```python
from build123d import *

# Parameters (mm, degrees)
SKETCH_1_W               = 35
SKETCH_1_H               = 25
EXTRUDE_1_DEPTH          = 8
FILLET_1_R               = 3
SKETCH_2_R               = 1.524999998
CUT_EXTRUDE_1_DEPTH      = 1
CUT_EXTRUDE_1_DEPTH_BACK = 9
SKETCH_3_R               = 3.099999998
CUT_EXTRUDE_2_DEPTH      = 4
HOLE_WIZARD_M4_1_D       = 3.3
HOLE_WIZARD_M4_2_D       = 3.3


with BuildPart() as part:
    # 草图1 → 凸台-拉伸1 (new body)
    with BuildSketch(Plane.XY):
        Rectangle(SKETCH_1_W, SKETCH_1_H)
    extrude(amount=EXTRUDE_1_DEPTH)

    # 圆角1
    fillet_1_edges = [part.edges().sort_by_distance(p)[0] for p in [
        (17.5, -12.5, 4),
        (-17.5, -12.5, 4),
        (-17.5, 12.5, 4),
        (17.5, 12.5, 4),
    ]]
    fillet(fillet_1_edges, radius=FILLET_1_R)

    # 草图2 → 切除-拉伸1 (cut, two sides)
    with BuildSketch(Plane.XY.offset(8)) as cut_extrude_1_sk:
        with Locations((3, 5.000000008)):
            Circle(SKETCH_2_R)
        with Locations((3, -4.999999992)):
            Circle(SKETCH_2_R)
        with Locations((-12, 5.000000008)):
            Circle(SKETCH_2_R)
        with Locations((-12, -4.999999992)):
            Circle(SKETCH_2_R)
    extrude(amount=CUT_EXTRUDE_1_DEPTH, mode=Mode.SUBTRACT)
    extrude(cut_extrude_1_sk.sketch, amount=-CUT_EXTRUDE_1_DEPTH_BACK, mode=Mode.SUBTRACT)

    # 草图3 → 切除-拉伸2 (cut)
    with BuildSketch(Plane.XY.offset(8)):
        with Locations((3, 5.000000008)):
            Circle(SKETCH_3_R)
        with Locations((-12, 5.000000008)):
            Circle(SKETCH_3_R)
        with Locations((3, -4.999999992)):
            Circle(SKETCH_3_R)
        with Locations((-12, -4.999999992)):
            Circle(SKETCH_3_R)
    extrude(amount=-CUT_EXTRUDE_2_DEPTH, mode=Mode.SUBTRACT)

    # M4 螺纹孔1 (through all)
    with Locations(Plane(origin=(-3.5, -12.5, 4), x_dir=(0, 0, -1), z_dir=(0, -1, 0))):
        with Locations((0, 0), (0, 15)):
            Hole(HOLE_WIZARD_M4_1_D / 2)

    # M4 螺纹孔2 (through all)
    with Locations(Plane.ZY.offset(17.5)):
        with Locations((4, 9e-09)):
            Hole(HOLE_WIZARD_M4_2_D / 2)


solid = part.part
```
For this review, take the finished solid that the model builds, in its own axes (mm). A direction names the side the tool comes from. Round coordinates to 2 decimals unless told otherwise and drop trailing zeros. Loops run counter-clockwise (first coordinate to the right, second up) from the corner with the lowest first, then second, coordinate; pieces in that order, holes last.
(1) Tool access review of faces 4 (the cylindrical face through (-15.1, -4.9, 6)), 5 (the flat face through (0, 0, 8)): name each direction out of +Z, -Z, +X, -X, +Y, -Y from which nothing blocks a thin tool from reaching the whole face with its end or side.
Returned:
face 4: +Z
face 5: +Z, +X, -X, +Y, -Y
(2) We need section B-B (x = 3). Give the boundary of the cut face in (y, z) (3 decimals), plus the area to 3 significant figures.
Returned:
outline: (-12.5, 0) - (-6.525, 0) - (-6.525, 4) - (-8.1, 4) - (-8.1, 8) - (-12.5, 8) - close; (-3.475, 0) - (3.475, 0) - (3.475, 4) - (1.9, 4) - (1.9, 8) - (-1.9, 8) - (-1.9, 4) - (-3.475, 4) - close; (6.525, 0) - (12.5, 0) - (12.5, 8) - (8.1, 8) - (8.1, 4) - (6.525, 4) - close; hole circle Ø3.3 at (0, 4)
area: 117 mm2
(3) We need section C-C (z = 4.75). State how many separate pieces and enclosed holes the cut face has, plus the area to 3 significant figures.
Returned:
separate pieces: 6
enclosed holes: 4
area: 514 mm2
(4) We need section A-A (y = 5). Give the boundary of the cut face in (x, z) (3 decimals), plus the area to 3 significant figures.
Returned:
outline: (-17.5, 0) - (-13.525, 0) - (-13.525, 4) - (-15.1, 4) - (-15.1, 8) - (-17.5, 8) - close; (-10.475, 0) - (1.475, 0) - (1.475, 4) - (-0.1, 4) - (-0.1, 8) - (-8.9, 8) - (-8.9, 4) - (-10.475, 4) - close; (4.525, 0) - (17.5, 0) - (17.5, 8) - (6.1, 8) - (6.1, 4) - (4.525, 4) - close; hole circle Ø3.3 at (-3.5, 4); hole circle Ø3.3 at (11.5, 4)
area: 189 mm2
(5) Wall thickness on line 1 along Y through (x, z) = (3, 5.75); line 2 along X through (y, z) = (11.25, 5.5); line 3 along X through (y, z) = (3.25, 3.75): over which ranges is each line inside the solid? List them lowest first.
Returned:
line 1: y = -12.5 to -8.1, -1.9 to 1.9, 8.1 to 12.5
line 2: x = -16.94 to -4.19, -2.81 to 10.81, 12.19 to 16.94
line 3: x = -17.5 to -5.13, -1.87 to 9.87, 13.13 to 17.5
(6) Mouldability with a two-part tool opening along Z and no side actions: class faces 1 (the cylindrical face through (-10.402, 0.496, 2.426)), 2 (the flat face through (0, 0, 0)), 3 (the flat face through (17.5, 0, 2)) as released by +Z, released by -Z, zero draft, split by the parting line, or undercut.
Returned:
face 1: undercut
face 2: released by -Z
face 3: zero draft
(7) We need section D-D (x = 6.5). Give the boundary of the cut face in (y, z), plus the area to 3 significant figures.
Returned:
outline: (-12.5, 0) - (12.5, 0) - (12.5, 8) - (-12.5, 8) - close; hole circle Ø3.3 at (0, 4)
area: 191 mm2
(8) Clearance check with flat-ended pins moving along their axes: P1, Ø2.5, axis at x = 3, y = -5, coming from the +Z side; P2, Ø1.9, axis at x = -13, y = -5, coming from the +Z side. State where each tip first meets the part, or that it passes through.
Returned:
P1: passes through
P2: stops at z = 4
